Answer from the drawing. Dimensions are ordinates in mm from the lowest x, y and z of the part. A direction names the side the tool comes from. Coordinates: 2 decimals unless noted, no trailing zeros. Write each loop counter-clockwise with the first axis right and the second up, starting at its lowest first coordinate (ties: lowest second). Pieces come first, ordered by that corner, then holes.
(1) Which of the six approach directions +Z, -Z, +X, -X, +Y, -Y give full straight-line access (tool end or side, diameter ignored) to the marked faces 4 and 5?
(2) Find the intervals of material crossed by probe 1 along X at (y, z) = (12.7, 8.75); probe 2 along X at (y, z) = (12.7, 0.85); probe 3 along Y at (x, z) = (9, 4.75), in increasing order.
(3) Given pin 1 (3 mm diameter, centred on y = 9.5, z = 2, fed in from +X); pin 2 (1.5 mm diameter, centred on x = 33.5, y = 17.5, fed in from -Z); pin 3 (5 mm diameter, centred on x = 32, y = 14, fed in from +Z); pin 4 (2 mm diameter, centred on x = 20, z = 1.5, fed in from +Y), each flat-ended and moving along its own axis, determine where each tip first touches the part or whether it passes through.
(4) The mould has two halves that part along X. Classify the marked faces 1, 2 and 3: +X half, -X half, draft (parallel to the pull), parting line (faces both ways), or undercut.
(5) Section A-A on x = 31.75 is taken. Write down the section's boundary in (y, z), then the cut area to 3 significant figures.
(6) Section C-C on z = 11 is taken. Write down the section's boundary in (x, y).
(7) Section B-B on y = 12.7 is taken. Write down the section's boundary in (x, z), then the cut area to 3 significant figures.
(8) Section D-D on y = 9.5 is taken. Write down the section's boundary in (x, z), then the cut area to 3 significant figures.
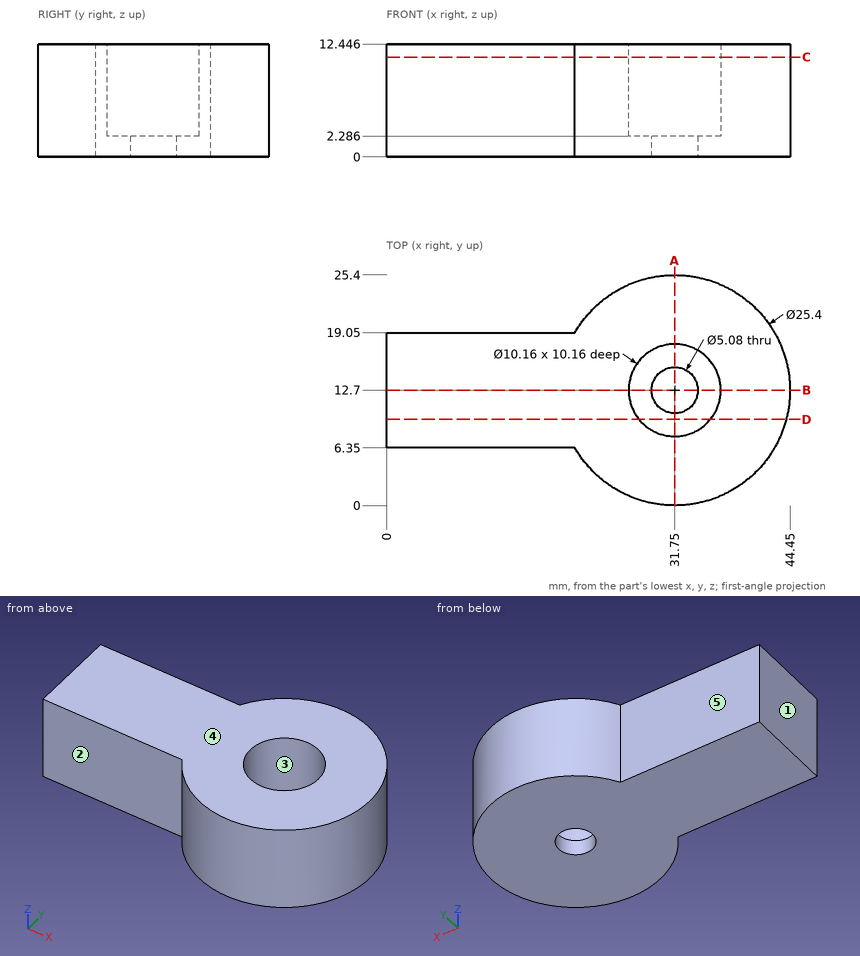
Response:
1. face 4: +Z, +X, -X, +Y, -Y
1. face 5: +Z, -Z, -X, +Y
2. probe 1: x = 0 to 26.67, 36.83 to 44.45
2. probe 2: x = 0 to 29.21, 34.29 to 44.45
2. probe 3: y = 6.35 to 19.05
3. pin 1: stops at x = 44.34
3. pin 2: stops at z = 0
3. pin 3: stops at z = 2.29
3. pin 4: stops at y = 19.46
4. face 1: -X half
4. face 2: draft
4. face 3: undercut
5. outline: (0, 0) - (10.16, 0) - (10.16, 2.29) - (7.62, 2.29) - (7.62, 12.45) - (0, 12.45) - close; (15.24, 0) - (25.4, 0) - (25.4, 12.45) - (17.78, 12.45) - (17.78, 2.29) - (15.24, 2.29) - close
5. area: 201 mm2
6. outline: (0, 6.35) - (20.75, 6.35) arc R12.7 ccw (long way) to (20.75, 19.05) - (0, 19.05) - close; hole circle Ø10.16 at (31.75, 12.7)
7. outline: (0, 0) - (29.21, 0) - (29.21, 2.29) - (26.67, 2.29) - (26.67, 12.45) - (0, 12.45) - close; (34.29, 0) - (44.45, 0) - (44.45, 12.45) - (36.83, 12.45) - (36.83, 2.29) - (34.29, 2.29) - close
7. area: 438 mm2
8. outline: (0, 0) - (44.04, 0) - (44.04, 12.45) - (35.7, 12.45) - (35.7, 2.29) - (27.8, 2.29) - (27.8, 12.45) - (0, 12.45) - close
8. area: 468 mm2
